Can you work these out from the model? Positions are in its coordinate system, mm. Face numbers are marked on the shaded views. A direction names the side the tool comes from. Coordinates: 2 decimals unless noted, no trailing zeros. Write each loop counter-clockwise with the first axis right and the second up, starting at its lowest first coordinate (ties: lowest second). Pieces come first, ordered by that corner, then holes. Notation, with made-up numbers: (-9, -34) - (37, -34) arc R19 ccw to (37, -7) - close; hole circle Ø8 at (59.5, 3). An arc over 180 degrees is marked (long way). Use one line per item in the form item = value. Start each with the question number.
(1) If we section it at A-A on z = -61: Please give me the cut outline in (x, y) (3 decimals), then the cut area to 3 significant figures.
(2) If we section it at D-D on x = -5: Please give me the cut outline in (y, z), then the cut area to 3 significant figures.
(3) For pin 1 Ø6 at (x, y) = (2.5, -3.5) entering from +Z; pin 2 Ø1.5 at (y, z) = (-2, -19) entering from -X; pin 3 Ø1.5 at (x, z) = (-1.5, -34.5) entering from +Y; pin 4 Ø6 at (x, y) = (-1, -1) entering from +Z, each with a flat end and sliding along its axis, tell me the tip position at first contact or that it passes through.
(4) On a 3-axis mill with a long thin cutter (end or side, diameter ignored), from which of +Z, -Z, +X, -X, +Y, -Y can I reach the whole of each face in a straight line? I mean the marked faces 1 and 2. Say none if no direction works.
(5) If we section it at B-B on x = 3: Please give me the cut outline in (y, z).
(6) If I drill on probe 1 along Y at (x, z) = (1.25, -57); probe 2 along Z at (x, y) = (-1.75, 4.5); probe 3 along X at (y, z) = (-0.5, -48), over which ranges is the centre line in solid material (lowest first)? Write a range as from..to.
(7) If we section it at C-C on y = -2: Please give me the cut outline in (x, z), then the cut area to 3 significant figures.
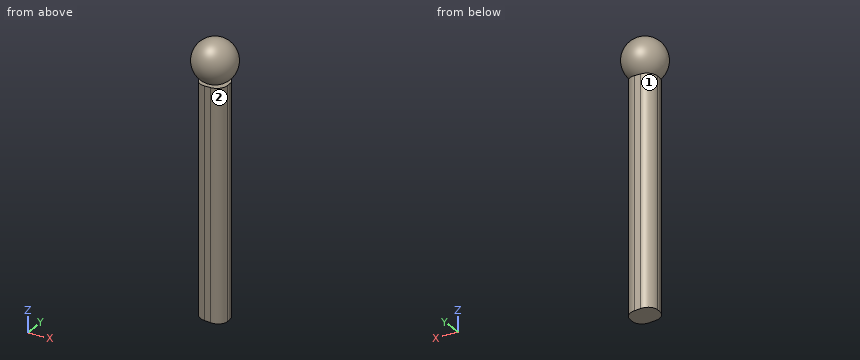
```python
from build123d import *

# Parameters (mm, degrees)
F3_DEPTH      = 3.81
F3_DEPTH_BACK = 3.81
F4_R          = 3.175


with BuildPart() as f1:
    # F0 (on Front) → F1 (revolve)
    with BuildSketch(Plane.XZ):
        with BuildLine():
            Line((0, -6.35), (0, 6.35))
            ThreePointArc((0, 6.35), (-6.35, 0), (0, -6.35))
        make_face()
    revolve(axis=Axis((0, 0, 0), (0, 0, -1)))

    # F2 (on Front) → F3 (join, two sides)
    with BuildSketch(Plane.XZ) as f3_sk:
        Polygon((4.1104733182, -5.9445748625), (-4.1104737839, -5.9445748625), (-4.1104737839, -74.5245748625), (4.1104733182, -75.1735985691), align=None)
    extrude(amount=-F3_DEPTH)
    extrude(f3_sk.sketch, amount=F3_DEPTH_BACK)

    # F4
    f4_edges = [f1.edges().sort_by_distance(p)[0] for p in [
        (4.110473, -3.81, -40.559087),
        (4.110473, 3.81, -40.559087),
        (-4.110474, -3.81, -40.234575),
        (-4.110474, 3.81, -40.234575),
    ]]
    fillet(f4_edges, radius=F4_R)


solid = f1.part
```
Reported:
q1.outline = (-4.11, -0.635) arc R3.175 ccw to (-0.935, -3.81) - (0.935, -3.81) arc R3.175 ccw to (4.11, -0.635) - (4.11, 0.635) arc R3.175 ccw to (0.935, 3.81) - (-0.935, 3.81) arc R3.175 ccw to (-4.11, 0.635) - close
q1.area = 54.0 mm2
q2.outline = circle Ø7.83 at (0, 0)
q2.area = 48.1 mm2
q3.pin_1 = 6.22
q3.pin_2 = -4.05
q3.pin_3 = 3.81
q3.pin_4 = 6.35
q4.face_1 = -Z, -X, +Y
q4.face_2 = -Z, +X, -Y
q5.outline = circle Ø11.19 at (0, 0); (-3.05, -75.09) - (3.05, -75.09) - (3.05, -5.94) - (-3.05, -5.94) - close
q6.probe_1 = -3.79..3.79
q6.probe_2 = -4.12..4.12
q6.probe_3 = -4.11..4.11
q7.outline = (-3.8, -74.55) - (3.8, -75.15) - (3.8, -5.94) - (0.99, -5.94) arc R6.03 ccw (long way) to (-0.99, -5.94) - (-3.8, -5.94) - close
q7.area = 638 mm2
